Input: part model. Units: mm. Frame: model coordinates. A direction names the side the tool comes from. Round coordinates to 2 decimals unless told otherwise and drop trailing zeros. Loops run counter-clockwise (first coordinate to the right, second up) from the corner with the lowest first, then second, coordinate; pieces in that order, holes last. Notation, with made-up numbers: (89, 70.25) -> (107, 70.25) arc R20 cw to (107, 96.25) -> close; hole circle Ø8 at (-29, 21.25). An arc over 180 degrees is marked (long way). Answer as a JSON object with one key per item and string values. Group by question number.
Item 1: Set-up query: faces 1 (the flat face through (-196.04, 3.13, 36.7)), 2 (the flat face through (-25, 3, -19.05)). Return all of +Z, -Z, +X, -X, +Y, -Y with unobstructed straight access to the full face (end or side cutting, diameter ignored); none if empty.
Item 2: Pin query (flat end, axial travel): pin 1 (1.9 mm diameter, centred on x = -144.5, y = 4, fed in from -Z); pin 2 (1.9 mm diameter, centred on x = -60.5, y = 2, fed in from -Z); pin 3 (2 mm diameter, centred on y = 3, z = 11, fed in from -X). Return the tip coordinate at first contact, or that it passes through.
Item 3: Section query A-A on x = -25. Return loops of the section in (y, z) (3 decimals), and give its area (3 significant figures).
Item 4: Material intervals for line 1 (X direction, y = 4.5, z = 0) (3 decimals); line 2 (X direction, y = 4.5, z = 6.5) (3 decimals); line 3 (Z direction, x = -144, y = 2.5), sorted ascending. Write a range as [from, to].
Item 5: Section query B-B on x = -72.5. Return loops of the section in (y, z).
Item 6: Section query C-C on y = 4.75. Count the separate pieces of the cut face and the enclosed holes in it, and give its area (3 significant figures).
Item 7: Draft query along Z for faces 3 (the cylindrical face through (26.514, 3.219, 13.49)), 4 (the flat face through (-170, 3, -2)), 5 (the cylindrical face through (-104.91, 3.22, 25.66)), 6 (the flat face through (28.325, 3, 0)). Return one class per face: released by +Z, released by -Z, zero draft, split by the parting line, or undercut.
from build123d import *

# Parameters (mm, degrees)
CROQUIS1_R              = 6.35
SALIENTE_EXTRUIR1_DEPTH = 6.35
CORTAR_EXTRUIR2_DEPTH   = 225.270156497
CORTAR_EXTRUIR3_DEPTH   = 225.270156497
REDONDEO1_R             = 10
CROQUIS8_R              = 2.38125
CORTAR_EXTRUIR4_DEPTH   = 225.270156497
REDONDEO2_R             = 6.35
CROQUIS10_R             = 3.175
CORTAR_EXTRUIR6_DEPTH   = 225.270156497


with BuildPart() as part:
    # Croquis1 → Saliente-Extruir1 (new body)
    with BuildSketch(Plane(origin=(0, 0, 0), x_dir=(1, 0, 0), z_dir=(0, 1, 0))):
        with BuildLine():
            Line((37.5, -25.4), (52.5, 0))
            Line((52.5, 0), (37.5, 25.4))
            Line((37.5, 25.4), (-105, 25.4))
            Line((-105, 25.4), (-149.746813481, 47.731727951))
            ThreePointArc((-149.746813481, 47.731727951), (-154.357530471, 48.146831931), (-158.024774803, 45.321528145))
            Line((-158.024774803, 45.321528145), (-170, 25.4))
            Line((-170, 25.4), (-170, -25.4))
            Line((-170, -25.4), (-218.893171651, -46.613192851))
            Line((-218.893171651, -46.613192851), (-152.75365104, -48.397689977))
            ThreePointArc((-152.75365104, -48.397689977), (-151.209247261, -48.24975741), (-149.746813481, -47.731727951))
            Line((-149.746813481, -47.731727951), (-105, -25.4))
            Line((-105, -25.4), (37.5, -25.4))
        make_face()
        with Locations(Location((-155, 0, 0), (0, 0, 270))):
            Circle(CROQUIS1_R, mode=Mode.SUBTRACT)
        with Locations(Location((-25, 0, 0), (0, 0, 270))):
            Circle(CROQUIS1_R, mode=Mode.SUBTRACT)
        with BuildLine():
            Line((-129.045100716, 30.303281185), (-147.329198773, 39.428299747))
            ThreePointArc((-147.329198773, 39.428299747), (-151.939915763, 39.843403727), (-155.607160095, 37.018099941))
            Line((-155.607160095, 37.018099941), (-161.092389512, 27.893081378))
            ThreePointArc((-161.092389512, 27.893081378), (-161.177056347, 21.495189828), (-155.65, 18.271553233))
            Line((-155.65, 18.271553233), (-131.880672526, 18.271553233))
            ThreePointArc((-131.880672526, 18.271553233), (-125.699998109, 23.164925706), (-129.045100716, 30.303281185))
        make_face(mode=Mode.SUBTRACT)
        with BuildLine():
            Line((-129.045100716, -30.303281185), (-147.329198773, -39.428299747))
            ThreePointArc((-147.329198773, -39.428299747), (-151.939915763, -39.843403727), (-155.607160095, -37.018099941))
            Line((-155.607160095, -37.018099941), (-161.092389512, -27.893081378))
            ThreePointArc((-161.092389512, -27.893081378), (-161.177056347, -21.495189828), (-155.65, -18.271553233))
            Line((-155.65, -18.271553233), (-131.880672526, -18.271553233))
            ThreePointArc((-131.880672526, -18.271553233), (-125.699998109, -23.164925706), (-129.045100716, -30.303281185))
        make_face(mode=Mode.SUBTRACT)
    extrude(amount=SALIENTE_EXTRUIR1_DEPTH)

    # Croquis5 → Cortar-Extruir2 (cut, through all)
    with BuildSketch(Plane(origin=(0, 6.35, 0), x_dir=(1, 0, 0), z_dir=(0, 1, 0))):
        with BuildLine():
            Line((-44.05, 22.225), (-5.95, 22.225))
            ThreePointArc((-5.95, 22.225), (-4.3625, 20.6375), (-5.95, 19.05))
            Line((-5.95, 19.05), (-44.05, 19.05))
            ThreePointArc((-44.05, 19.05), (-45.6375, 20.6375), (-44.05, 22.225))
        make_face()
        with BuildLine():
            Line((-5.95, -19.05), (-44.05, -19.05))
            ThreePointArc((-44.05, -19.05), (-45.6375, -20.6375), (-44.05, -22.225))
            Line((-44.05, -22.225), (-5.95, -22.225))
            ThreePointArc((-5.95, -22.225), (-4.3625, -20.6375), (-5.95, -19.05))
        make_face()
    extrude(amount=-CORTAR_EXTRUIR2_DEPTH, mode=Mode.SUBTRACT)

    # Croquis7 → Cortar-Extruir3 (cut, through all)
    with BuildSketch(Plane(origin=(0, 6.35, 0), x_dir=(1, 0, 0), z_dir=(0, 1, 0))):
        with BuildLine():
            Line((-78.775, 15.4), (-51.475, 15.4))
            ThreePointArc((-51.475, 15.4), (-46.984871939, 13.540128061), (-45.125, 9.05))
            Line((-45.125, 9.05), (-45.125, -9.05))
            ThreePointArc((-45.125, -9.05), (-46.984871939, -13.540128061), (-51.475, -15.4))
            Line((-51.475, -15.4), (-78.775, -15.4))
            ThreePointArc((-78.775, -15.4), (-83.265128061, -13.540128061), (-85.125, -9.05))
            Line((-85.125, -9.05), (-85.125, 9.05))
            ThreePointArc((-85.125, 9.05), (-83.265128061, 13.540128061), (-78.775, 15.4))
        make_face()
        with BuildLine():
            Line((9.675, 15.4), (21.975, 15.4))
            ThreePointArc((21.975, 15.4), (26.465128061, 13.540128061), (28.325, 9.05))
            Line((28.325, 9.05), (28.325, -9.05))
            ThreePointArc((28.325, -9.05), (26.465128061, -13.540128061), (21.975, -15.4))
            Line((21.975, -15.4), (9.675, -15.4))
            ThreePointArc((9.675, -15.4), (5.184871939, -13.540128061), (3.325, -9.05))
            Line((3.325, -9.05), (3.325, 9.05))
            ThreePointArc((3.325, 9.05), (5.184871939, 13.540128061), (9.675, 15.4))
        make_face()
    extrude(amount=-CORTAR_EXTRUIR3_DEPTH, mode=Mode.SUBTRACT)

    # Redondeo1
    redondeo1_edges = [part.edges().sort_by_distance(p)[0] for p in [
        (-105, 3.175, 25.4),
        (-105, 3.175, -25.4),
    ]]
    fillet(redondeo1_edges, radius=REDONDEO1_R)

    # Croquis8 → Cortar-Extruir4 (cut, through all)
    with BuildSketch(Plane(origin=(0, 6.35, 0), x_dir=(1, 0, 0), z_dir=(0, 1, 0))):
        with Locations(Location((-93.125, 0, 0), (0, 0, 270))):
            Circle(CROQUIS8_R)
        with Locations(Location((-93.125, 19.4, 0), (0, 0, 270))):
            Circle(CROQUIS8_R)
        with Locations(Location((-93.125, -19.4, 0), (0, 0, 270))):
            Circle(CROQUIS8_R)
    extrude(amount=-CORTAR_EXTRUIR4_DEPTH, mode=Mode.SUBTRACT)

    # Redondeo2
    redondeo2_edges = [part.edges().sort_by_distance(p)[0] for p in [
        (-170, 3.175, 25.4),
    ]]
    fillet(redondeo2_edges, radius=REDONDEO2_R)

    # Croquis10 → Cortar-Extruir6 (cut, through all)
    with BuildSketch(Plane(origin=(0, 6.35, 0), x_dir=(1, 0, 0), z_dir=(0, 1, 0))):
        with Locations(Location((-117.61165924, -10, 0), (0, 0, 270))):
            Circle(CROQUIS10_R)
        with Locations(Location((-117.61165924, 10, 0), (0, 0, 270))):
            Circle(CROQUIS10_R)
    extrude(amount=-CORTAR_EXTRUIR6_DEPTH, mode=Mode.SUBTRACT)


solid = part.part
Solved:
{
 "1": {"face 1": "-Z, -X, +Y, -Y", "face 2": "+Y, -Y"},
 "2": {"pin 1": "z = -45.59", "pin 2": "z = -25.4", "pin 3": "x = -170"},
 "3": {"outline": "(0, -25.4) -> (6.35, -25.4) -> (6.35, -22.225) -> (0, -22.225) -> close; (0, -19.05) -> (6.35, -19.05) -> (6.35, -6.35) -> (0, -6.35) -> close; (0, 6.35) -> (6.35, 6.35) -> (6.35, 19.05) -> (0, 19.05) -> close; (0, 22.225) -> (6.35, 22.225) -> (6.35, 25.4) -> (0, 25.4) -> close", "area": "202 mm²"},
 "4": {"line 1": "[-170, -161.35], [-148.65, -95.506], [-90.744, -85.125], [-45.125, -31.35], [-18.65, 3.325], [28.325, 52.5]", "line 2": "[-170, -85.125], [-45.125, 3.325], [28.325, 48.661]", "line 3": "[-44.86, -37.77], [-18.27, 18.27], [37.77, 44.86]"},
 "5": {"outline": "(0, -25.4) -> (6.35, -25.4) -> (6.35, -15.4) -> (0, -15.4) -> close; (0, 15.4) -> (6.35, 15.4) -> (6.35, 25.4) -> (0, 25.4) -> close"},
 "6": {"separate pieces": "1", "enclosed holes": "13", "area": "9,510 mm²"},
 "7": {"face 3": "undercut", "face 4": "zero draft", "face 5": "released by +Z", "face 6": "undercut"}
}
